Design review of the part built by this model. Coordinates are the model's own, in mm. Face numbers are marked on the shaded views. A direction names the side the tool comes from. Give positions to 0.01 mm unless a question says otherwise; leave off trailing zeros. Write each loop counter-clockwise with the first axis right and the second up, starting at its lowest first coordinate (ties: lowest second). Pieces come first, ordered by that corner, then holes. Notation, with made-up numbers: (-38.75, 20) -> (-32.75, 20) arc R21 cw to (-32.75, 38) -> close; hole circle Ø9 at (-22, 29). An arc over 180 degrees is marked (long way). Write each question's results on one line, items separated by ' | '. Start each with the question number.
(1) Take a section at A-A (z = 11.5). State the section outline as (x, y) points, plus the area to 3 significant figures.
(2) Take a section at B-B (y = -53). State the section outline as (x, z) points (3 decimals).
(3) Take a section at C-C (x = 38). State the section outline as (y, z) points, plus the area to 3 significant figures.
(4) Take a section at D-D (y = -65). State the section outline as (x, z) points (3 decimals), plus the area to 3 significant figures.
(5) For the marked faces 1, 2 and 3, list the 3-axis set-ups (+Z, -Z, +X, -X, +Y, -Y) from which the entire face can be reached by the end or side of a thin tool; tool diameter is ignored.
(6) Clearance check with flat-ended pins moving along their axes: pin 1 (12 mm diameter, centred on y = -84, z = 62.5, fed in from +X); pin 2 (4 mm diameter, centred on y = -74, z = 77, fed in from -X); pin 3 (8 mm diameter, centred on x = -6.5, y = -74, fed in from +Z). State where each tip first meets the part, or that it passes through.
(7) To check wall thickness, follow probe 1 along Z at (x, y) = (20.5, -62.5); probe 2 along Y at (x, z) = (33.5, 44); probe 3 along Y at (x, z) = (-37, 86). State the ranges of each line that lie inside material, in increasing order.
(8) Mouldability with a two-part tool opening along X and no side actions: class the marked faces 4, 5 and 6 as released by +X, released by -X, zero draft, split by the parting line, or undercut.
from build123d import *

# Parameters (mm, degrees)
F0_W      = 50.8
F0_H      = 101.6
F1_DEPTH  = 101.6
F4_DEPTH  = 101.6
F5_T      = -3.81
F6_W      = 3.81
F6_H      = 101.6
F7_DEPTH  = 101.6
F8_DEPTH  = 25.4
F9_W      = 50.8
F9_H      = 5.08
F10_DEPTH = 63.5
F11_W     = 46.99
F11_H     = 3.81
F12_DEPTH = 25.4
F13_DEPTH = 101.6
F14_DEPTH = 25.4
F15_W     = 1.905
F15_H     = 25.4
F16_DEPTH = 57.15
F18_W     = 3.81
F18_H     = 97.79
F19_DEPTH = 49.53


with BuildPart() as f1:
    # F0 (on Top) → F1 (new body)
    with BuildSketch(Plane.XY):
        with Locations((25.4, -50.8)):
            Rectangle(F0_W, F0_H)
    extrude(amount=F1_DEPTH)

    # F2 (on face) → F4 (join)
    with BuildSketch(Plane.XY.offset(101.6)):
        with BuildLine():
            Line((50.8, 0), (50.8, -101.6))
            ThreePointArc((50.8, -101.6), (101.6, -50.8), (50.8, 0))
        make_face()
    extrude(amount=-F4_DEPTH)

    # F5
    f5_openings = [f1.faces().sort_by_distance(p)[0] for p in [
        (46.057827, -50.8, 101.6),
    ]]
    offset(amount=F5_T, openings=f5_openings)

    # F6 (on face) → F7 (join)
    with BuildSketch(Plane.XZ.offset(101.6)):
        with Locations((48.895, 50.8)):
            Rectangle(F6_W, F6_H)
    extrude(amount=-F7_DEPTH)

    # F8 (cut): a face of the model
    f8_faces = [f1.faces().sort_by_distance(p)[0] for p in [
        (3.81, -50.8, 52.705),
    ]]
    extrude(f8_faces, amount=-F8_DEPTH, mode=Mode.SUBTRACT)

    # F9 (on face) → F10 (join)
    with BuildSketch(Plane.XZ.offset(101.6)):
        with Locations((25.4, 73.9570113206)):
            Rectangle(F9_W, F9_H)
    extrude(amount=-F10_DEPTH)

    # F11 (on face) → F12 (join)
    with BuildSketch(Plane.XY.offset(76.4970113206)):
        with Locations((23.495, -40.005)):
            Rectangle(F11_W, F11_H)
    extrude(amount=F12_DEPTH)

    # F13 (add): a face of the model
    f13_faces = [f1.faces().sort_by_distance(p)[0] for p in [
        (23.495, -40.005, 101.8970113206),
    ]]
    extrude(f13_faces, amount=-F13_DEPTH)

    # F14 (cut): a face of the model
    f14_faces = [f1.faces().sort_by_distance(p)[0] for p in [
        (23.495, -97.79, 37.6135056603),
    ]]
    extrude(f14_faces, amount=-F14_DEPTH, mode=Mode.SUBTRACT)

    # F15 (on face) → F16 (join)
    with BuildSketch(Plane.XZ.offset(41.91)):
        with Locations((0.9525, 89.1970113206)):
            Rectangle(F15_W, F15_H)
    extrude(amount=F16_DEPTH)

    # F17: F1 across plane


with BuildPart() as f1_1:
    add(f1.part)
    add(f1.part.mirror(Plane.YZ))

    # F18 (on face) → F19 (join)
    with BuildSketch(Plane(origin=(-50.8, 0, 0), x_dir=(0, -1, 0), z_dir=(-1, 0, 0))):
        with Locations((48.895, 52.705)):
            Rectangle(F18_W, F18_H)
    extrude(amount=F19_DEPTH)

    # F20: F1 across plane


with BuildPart() as f1_2:
    add(f1_1.part)
    add(f1_1.part.mirror(Plane.YZ))


solid = f1_2.part
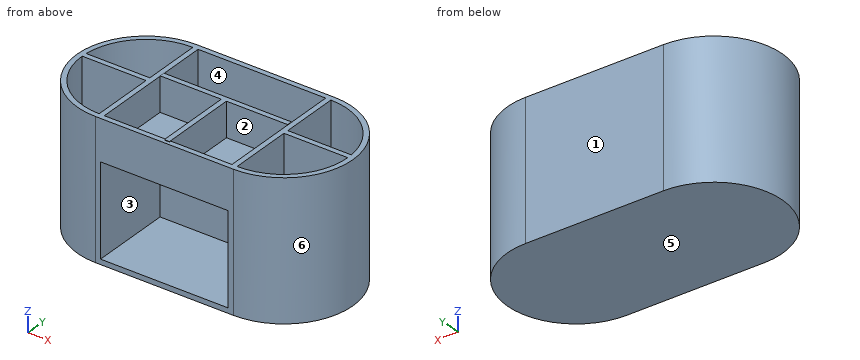
Report:
1) outline: (-50.8, -101.6) -> (-46.99, -101.6) -> (-46.99, -41.91) -> (46.99, -41.91) -> (46.99, -101.6) -> (50.8, -101.6) arc R50.8 ccw to (50.8, 0) -> (-50.8, 0) arc R50.8 ccw to start; hole (-97.79, -50.8) arc R46.99 ccw to (-50.8, -97.79) -> (-50.8, -50.8) -> close; hole (-97.64, -46.99) -> (-50.8, -46.99) -> (-50.8, -3.81) arc R46.99 ccw to start; hole (-46.99, -38.1) -> (46.99, -38.1) -> (46.99, -3.81) -> (-46.99, -3.81) -> close; hole (50.8, -97.79) arc R46.99 ccw to (97.79, -50.8) -> (50.8, -50.8) -> close; hole (50.8, -46.99) -> (97.64, -46.99) arc R46.99 ccw to (50.8, -3.81) -> close | area: 3,020 mm2
2) outline: (-101.552, 0) -> (101.552, 0) -> (101.552, 101.6) -> (97.738, 101.6) -> (97.738, 3.81) -> (50.8, 3.81) -> (50.8, 101.6) -> (46.99, 101.6) -> (46.99, 76.497) -> (1.905, 76.497) -> (1.905, 101.897) -> (-1.905, 101.897) -> (-1.905, 76.497) -> (-46.99, 76.497) -> (-46.99, 101.6) -> (-50.8, 101.6) -> (-50.8, 3.81) -> (-97.738, 3.81) -> (-97.738, 101.6) -> (-101.552, 101.6) -> close; hole (-46.99, 3.81) -> (46.99, 3.81) -> (46.99, 71.417) -> (-46.99, 71.417) -> close
3) outline: (-101.6, 0) -> (0, 0) -> (0, 101.6) -> (-3.81, 101.6) -> (-3.81, 3.81) -> (-38.1, 3.81) -> (-38.1, 101.9) -> (-41.91, 101.9) -> (-41.91, 76.5) -> (-97.79, 76.5) -> (-97.79, 101.6) -> (-101.6, 101.6) -> (-101.6, 71.42) -> (-41.91, 71.42) -> (-41.91, 3.81) -> (-101.6, 3.81) -> close | area: 1,530 mm2
4) outline: (-99.575, 0) -> (99.575, 0) -> (99.575, 101.6) -> (95.593, 101.6) -> (95.593, 3.81) -> (50.8, 3.81) -> (50.8, 101.6) -> (46.99, 101.6) -> (46.99, 76.497) -> (1.905, 76.497) -> (1.905, 101.897) -> (-1.905, 101.897) -> (-1.905, 76.497) -> (-46.99, 76.497) -> (-46.99, 101.6) -> (-50.8, 101.6) -> (-50.8, 3.81) -> (-95.593, 3.81) -> (-95.593, 101.6) -> (-99.575, 101.6) -> close; hole (-46.99, 3.81) -> (46.99, 3.81) -> (46.99, 71.417) -> (-46.99, 71.417) -> close | area: 2,860 mm2
5) face 1: +Z, -Z, +X, -X, +Y | face 2: +Z | face 3: -Y
6) pin 1: x = 93.7 | pin 2: x = -96.96 | pin 3: z = 76.5
7) probe 1: 0 to 3.81, 71.42 to 76.5 | probe 2: -41.91 to -38.1, -3.81 to 0 | probe 3: -101.6 to -97.79, -41.91 to -38.1, -3.81 to 0
8) face 4: undercut | face 5: zero draft | face 6: released by +X
